from build123d import *

# Parameters (mm, degrees)
BOSS_EXTRUDE1_DEPTH = 6
SKETCH3_W           = 6
SKETCH3_H           = 50
BOSS_EXTRUDE2_DEPTH = 6
LPATTERN1_COUNT     = 2
LPATTERN1_PITCH     = 206
SKETCH4_W           = 40
SKETCH4_H           = 6
SKETCH4_W_2         = 20
BOSS_EXTRUDE3_DEPTH = 6
SKETCH5_W           = 25
SKETCH5_H           = 10
CUT_EXTRUDE1_DEPTH  = 10


with BuildPart() as part:
    # Sketch1 → Boss-Extrude1 (new body)
    with BuildSketch(Plane.XY):
        with BuildLine():
            Line((-178, 100), (-178, 155))
            Line((-178, 155), (-200, 155))
            Line((-200, 155), (-200, 0))
            Line((-200, 0), (0, 0))
            Line((0, 0), (0, 155))
            Line((0, 155), (-22, 155))
            Line((-22, 155), (-22, 100))
            ThreePointArc((-22, 100), (-31.037807258, 63.555302549), (-56.056819802, 35.55625))
            ThreePointArc((-56.056819802, 35.55625), (-100, 17.5), (-143.943180198, 35.55625))
            ThreePointArc((-143.943180198, 35.55625), (-168.962192742, 63.555302549), (-178, 100))
        make_face()
    extrude(amount=BOSS_EXTRUDE1_DEPTH)

    # Sketch3 → Boss-Extrude2 (add)
    with BuildSketch(Plane.XY.offset(6)):
        with Locations((-203, 130)):
            Rectangle(SKETCH3_W, SKETCH3_H)
    boss_extrude2 = extrude(amount=-BOSS_EXTRUDE2_DEPTH)

    # LPattern1: Boss-Extrude2 ×2
    with Locations(*[(i * LPATTERN1_PITCH, 0, 0) for i in range(1, LPATTERN1_COUNT)]):
        add(boss_extrude2)

    # Sketch4 → Boss-Extrude3 (add)
    with BuildSketch(Plane.XY.offset(6)):
        with Locations((-180, -3)):
            Rectangle(SKETCH4_W, SKETCH4_H)
        with Locations((-100, -3)):
            Rectangle(SKETCH4_W_2, SKETCH4_H)
        with Locations((-20, -3)):
            Rectangle(SKETCH4_W, SKETCH4_H)
    extrude(amount=-BOSS_EXTRUDE3_DEPTH)

    # Sketch5 → Cut-Extrude1 (cut)
    with BuildSketch(Plane.XY.offset(6)):
        with Locations((-147.5, 5)):
            Rectangle(SKETCH5_W, SKETCH5_H)
    extrude(amount=-CUT_EXTRUDE1_DEPTH, mode=Mode.SUBTRACT)


solid = part.part
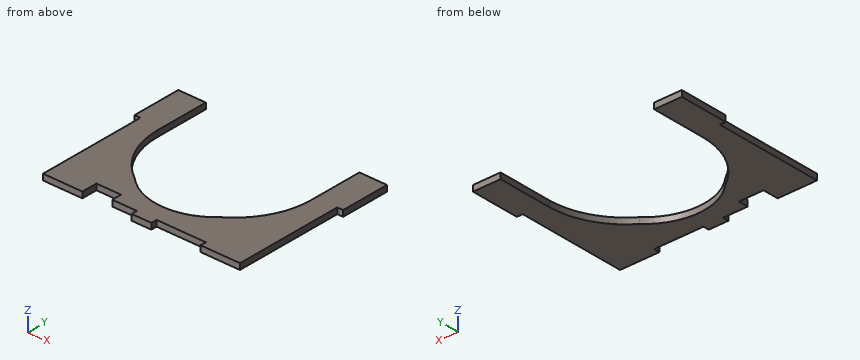
Geometry: final body of the model. Coordinates: model frame, mm. Round coordinates to 2 decimals unless told otherwise and drop trailing zeros. Order: outer loops, then holes, each group sorted by start corner. A loop starts at its lowest first (then second) coordinate and runs counter-clockwise, first axis right, second up. Notation, with made-up numbers: (-35, 25) -> (-10, 25) arc R24 cw to (-10, 63) -> close; hole circle Ø9 at (-16, -22). An arc over 180 degrees is marked (long way). Put each result on its own line as item: value. Start each with the question number.
Q1. Section D-D on x = -70. Return the cut outline in (y, z).
Q2. Section B-B on z = 2.95. Return the cut outline in (x, y).
Q3. Line query: probe 1 along X at (y, z) = (108, 2.65); probe 2 along X at (y, z) = (100.5, 0.55); probe 3 along Y at (x, z) = (-102, 3.4). Output: solid intervals per line, ascending.
Q4. Section A-A on y = 118. Return the cut outline in (x, z), and give its area (3 significant figures).
Q5. First-contact query: pin 1 (3 mm diameter, centred on y = -4, z = 1.5, fed in from -X); pin 2 (3 mm diameter, centred on x = -203, z = 4, fed in from -Y); pin 3 (12 mm diameter, centred on x = -160.5, y = 62, fed in from +Z); pin 4 (1.8 mm diameter, centred on y = -3, z = 1.5, fed in from +X). Flat tips, straight axial feed; report the tip coordinate or a pass-through.
Q6. Section C-C on y = 22. Return the cut outline in (x, z), and give its area (3 significant figures).
Ans:
1. outline: (0, 0) -> (25.17, 0) -> (25.17, 6) -> (0, 6) -> close
2. outline: (-206, 105) -> (-200, 105) -> (-200, -6) -> (-160, -6) -> (-160, 10) -> (-135, 10) -> (-135, 0) -> (-110, 0) -> (-110, -6) -> (-90, -6) -> (-90, 0) -> (-40, 0) -> (-40, -6) -> (0, -6) -> (0, 105) -> (6, 105) -> (6, 155) -> (-22, 155) -> (-22, 100) arc R78 cw to (-56.06, 35.56) arc R62.5 cw to (-143.94, 35.56) arc R78 cw to (-178, 100) -> (-178, 155) -> (-206, 155) -> close
3. probe 1: x = -206 to -178, -22 to 6
3. probe 2: x = -200 to -178, -22 to 0
3. probe 3: y = -6 to 17.53
4. outline: (-206, 0) -> (-178, 0) -> (-178, 6) -> (-206, 6) -> close; (-22, 0) -> (6, 0) -> (6, 6) -> (-22, 6) -> close
4. area: 336 mm2
5. pin 1: stops at x = -200
5. pin 2: stops at y = 105
5. pin 3: passes through
5. pin 4: stops at x = 0
6. outline: (-200, 0) -> (-123.29, 0) -> (-123.29, 6) -> (-200, 6) -> close; (-76.71, 0) -> (0, 0) -> (0, 6) -> (-76.71, 6) -> close
6. area: 921 mm2
